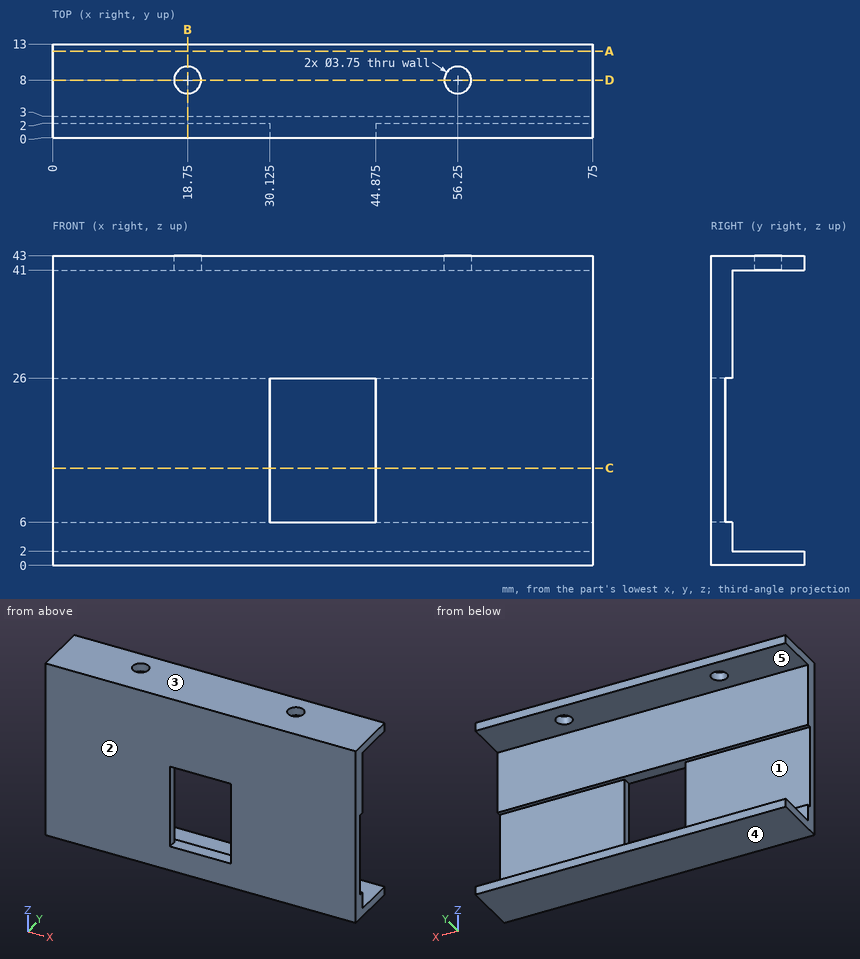
Here's the drawing with two shaded views (mm, measured from the low corner). I have some questions. A direction names the side the tool comes from. Round coordinates to 2 decimals unless told otherwise and drop trailing zeros. Write each loop counter-clockwise with the first axis right and the second up, starting at its lowest first coordinate (ties: lowest second). Pieces come first, ordered by that corner, then holes. Notation, with made-up numbers: M -4,13 L 54,13 A36 cw 54,51 Z; hole C 61,45 d10. An arc over 180 degrees is marked long. Write each question's results on one line, items separated by ' | '. Start each with the question number.
1. Imagine slicing it at B-B on x = 18.75. List the corners of the cut face in (y, z) for me (3 decimals).
2. On a 3-axis mill with a long thin cutter (end or side, diameter ignored), from which of +Z, -Z, +X, -X, +Y, -Y can I reach the whole of each face in a straight line? I mean the marked faces 4 and 5. Say none if no direction works.
3. Thinking about a two-plate mould opening in Z: for the marked faces 1, 2 and 3, which applies, +Z half, -Z half, draft (parallel to the pull), parting line (faces both ways), or undercut?
4. Imagine slicing it at C-C on z = 13.5. List the corners of the cut face in (x, y) for me (3 decimals).
5. Imagine slicing it at D-D on y = 8. List the corners of the cut face in (x, z) for me (3 decimals), and give its area (3 significant figures).
6. Imagine slicing it at A-A on y = 12. List the corners of the cut face in (x, z) for me.
7. I'm going to push flat-ended pins straight in: pin 1 Ø3 at (x, z) = (29, 5) entering from +Y; pin 2 Ø10 at (x, z) = (61.5, 15.5) entering from +Y. Where does each tip first touch, or does it pass through?
8. I need wall thicknesses on L1, parallel to Z at x = 56, y = 11.25; L2, parallel to X at y = 0.5, z = 8 (3 decimals); L3, parallel to Y at x = 56.25, z = 42.35 (3 decimals). Which ranges of each line are inside material? Lowest first, please. Write a range as from..to.
Result sheet:
1) outline: M 0,0 L 13,0 L 13,2 L 3,2 L 3,6 L 2,6 L 2,26 L 3,26 L 3,41 L 6.125,41 L 6.125,43 L 0,43 Z; M 9.875,41 L 13,41 L 13,43 L 9.875,43 Z
2) face 4: -Z, +X, -X, +Y, -Y | face 5: +X, -X, +Y
3) face 1: undercut | face 2: draft | face 3: +Z half
4) outline: M 0,0 L 30.125,0 L 30.125,2 L 0,2 Z; M 44.875,0 L 75,0 L 75,2 L 44.875,2 Z
5) outline: M 0,0 L 75,0 L 75,2 L 0,2 Z; M 0,41 L 16.875,41 L 16.875,43 L 0,43 Z; M 20.625,41 L 54.375,41 L 54.375,43 L 20.625,43 Z; M 58.125,41 L 75,41 L 75,43 L 58.125,43 Z | area: 285 mm^2
6) outline: M 0,0 L 75,0 L 75,2 L 0,2 Z; M 0,41 L 75,41 L 75,43 L 0,43 Z
7) pin 1: stops at y = 3 | pin 2: stops at y = 2
8) L1: z = 0..2, 41..43 | L2: x = 0..30.125, 44.875..75 | L3: y = 0..6.125, 9.875..13
